from build123d import *

# Parameters (mm, degrees)
SKETCH1_W           = 75
SKETCH1_H           = 18
BOSS_EXTRUDE1_DEPTH = 3
SKETCH2_W           = 8
SKETCH2_H           = 3
BOSS_EXTRUDE2_DEPTH = 3
SKETCH3_R           = 2.425
CUT_EXTRUDE1_DEPTH  = 3


with BuildPart() as part:
    # Sketch1 → Boss-Extrude1 (new body)
    with BuildSketch(Plane.XY):
        Rectangle(SKETCH1_W, SKETCH1_H)
    extrude(amount=BOSS_EXTRUDE1_DEPTH)

    # Sketch2 → Boss-Extrude2 (add)
    with BuildSketch(Plane(origin=(0, -9, 0), x_dir=(-1, 0, 0), z_dir=(0, -1, 0))):
        with Locations((-20.25, -1.5)):
            Rectangle(SKETCH2_W, SKETCH2_H)
        with Locations((0, -1.5)):
            Rectangle(SKETCH2_W, SKETCH2_H)
        with Locations((20.25, -1.5)):
            Rectangle(SKETCH2_W, SKETCH2_H)
    extrude(amount=BOSS_EXTRUDE2_DEPTH)

    # Sketch3 → Cut-Extrude1 (cut)
    with BuildSketch(Plane(origin=(0, 0, 0), x_dir=(-1, 0, 0), z_dir=(0, 0, -1))):
        with Locations((-28.5, 3.5)):
            Circle(SKETCH3_R)
        with Locations((28.5, 3.5)):
            Circle(SKETCH3_R)
        with Locations((-19.5, 3.5)):
            Circle(SKETCH3_R)
        with Locations((19.5, 3.5)):
            Circle(SKETCH3_R)
    extrude(amount=-CUT_EXTRUDE1_DEPTH, mode=Mode.SUBTRACT)


solid = part.part
The listing builds one solid part. Answer for the finished solid, in the listing's coordinates (mm). A direction names the side the tool comes from. Coordinates: 2 decimals unless noted, no trailing zeros. Loops run counter-clockwise (first coordinate to the right, second up) from the corner with the lowest first, then second, coordinate; pieces in that order, holes last.
1) Find section A-A on y = 3.5. Write down the section's boundary in (x, z) (3 decimals).
2) Find section B-B on x = -19.5. Write down the section's boundary in (y, z) (3 decimals), then the cut area to 4 significant figures.
3) Find section D-D on x = 5. Write down the section's boundary in (y, z), then the cut area to 3 significant figures.
4) Find the intervals of material crossed by L1, parallel to Y at x = -28.5, z = 2.4 (3 decimals); L2, parallel to X at y = -9.5, z = 0.5; L3, parallel to Y at x = 19.5, z = 2.35 (3 decimals), in increasing order.
5) Flat-ended cylindrical pins translate along their axes: pin 1 Ø0.9 at (x, z) = (-12.5, 2) entering from -Y; pin 2 Ø0.9 at (y, z) = (-10, 1) entering from +X; pin 3 Ø0.9 at (y, z) = (-10, 1) entering from -X. Find the tip coordinate at first contact, or state that the pin passes through.
6) Find section C-C on z = 0.65. Write down the section's boundary in (x, y) (3 decimals).
7) Determine the mould class of faces 1 (the face through (-4, -10, 2)), 2 (the face through (-37.5, 0, 1)), 3 (the face through (-1, 9, 1)) for opening direction X: pulls with the +X half, pulls with the -X half, needs draft (parallel to the pull), parting line crosses it, or undercut.
8) A tool of negligible diameter and unlimited length cuts with its end or side. For faces 4 (the face through (-26.077, 3.607, 1.479)), 5 (the face through (4, -10, 2)), 6 (the face through (-24.25, -10, 2)), 7 (the face through (24.25, -10, 2)), 8 (the face through (37.5, 0, 1)), from which of +Z, -Z, +X, -X, +Y, -Y can it reach the whole face along a straight path? Write none if from no direction.
Values:
1. outline: (-37.5, 0) - (-30.925, 0) - (-30.925, 3) - (-37.5, 3) - close; (-26.075, 0) - (-21.925, 0) - (-21.925, 3) - (-26.075, 3) - close; (-17.075, 0) - (17.075, 0) - (17.075, 3) - (-17.075, 3) - close; (21.925, 0) - (26.075, 0) - (26.075, 3) - (21.925, 3) - close; (30.925, 0) - (37.5, 0) - (37.5, 3) - (30.925, 3) - close
2. outline: (-12, 0) - (1.075, 0) - (1.075, 3) - (-12, 3) - close; (5.925, 0) - (9, 0) - (9, 3) - (5.925, 3) - close
2. area: 48.45 mm2
3. outline: (-9, 0) - (9, 0) - (9, 3) - (-9, 3) - close
3. area: 54.0 mm2
4. L1: y = -9 to 1.075, 5.925 to 9
4. L2: x = -24.25 to -16.25, -4 to 4, 16.25 to 24.25
4. L3: y = -12 to 1.075, 5.925 to 9
5. pin 1: stops at y = -9
5. pin 2: stops at x = 24.25
5. pin 3: stops at x = -24.25
6. outline: (-37.5, -9) - (-24.25, -9) - (-24.25, -12) - (-16.25, -12) - (-16.25, -9) - (-4, -9) - (-4, -12) - (4, -12) - (4, -9) - (16.25, -9) - (16.25, -12) - (24.25, -12) - (24.25, -9) - (37.5, -9) - (37.5, 9) - (-37.5, 9) - close; hole circle Ø4.85 at (-28.5, 3.5); hole circle Ø4.85 at (-19.5, 3.5); hole circle Ø4.85 at (19.5, 3.5); hole circle Ø4.85 at (28.5, 3.5)
7. face 1: undercut
7. face 2: pulls with the -X half
7. face 3: needs draft
8. face 4: +Z, -Z
8. face 5: +Z, -Z, -Y
8. face 6: +Z, -Z, -X, -Y
8. face 7: +Z, -Z, +X, -Y
8. face 8: +Z, -Z, +X, +Y, -Y
